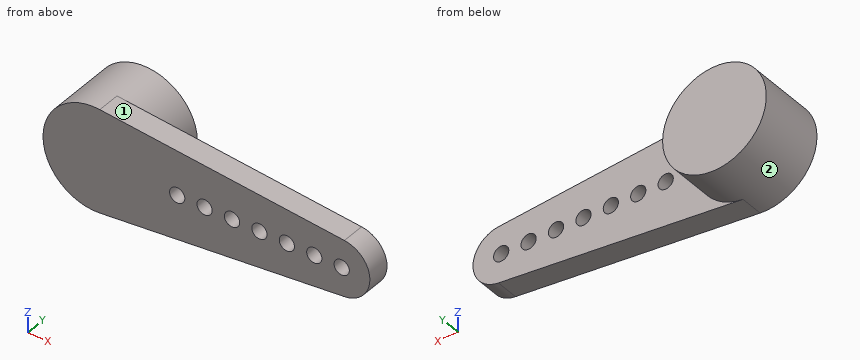
from build123d import *

# Parameters (mm, degrees)
SKETCH_1_R          = 3.405
EXTRUDE_1_DEPTH     = 4.5
EXTRUDE_2_DEPTH     = 1.52
SKETCH_3_R          = 0.5
CUT_EXTRUDE_1_DEPTH = 1.52


with BuildPart() as part:
    # 草图1 → 凸台-拉伸1 (new body)
    with BuildSketch(Plane(origin=(0, 0, 0), x_dir=(1, 0, 0), z_dir=(0, 1, 0))):
        Circle(SKETCH_1_R)
    extrude(amount=EXTRUDE_1_DEPTH)

    # 草图2 → 凸台-拉伸2 (add)
    with BuildSketch(Plane.XZ):
        with BuildLine():
            Line((0.326737118, 3.389287219), (16.38252237, 1.841462953))
            ThreePointArc((16.38252237, 1.841462953), (18.055, 0), (16.38252237, -1.841462953))
            Line((16.38252237, -1.841462953), (0.326737118, -3.389287219))
            ThreePointArc((0.326737118, -3.389287219), (-3.405, 0), (0.326737118, 3.389287219))
        make_face()
    extrude(amount=-EXTRUDE_2_DEPTH)

    # 草图3 → 切除-拉伸1 (cut)
    with BuildSketch(Plane.XZ):
        with Locations((16.205, 0)):
            Circle(SKETCH_3_R)
        with Locations((14.405, 0)):
            Circle(SKETCH_3_R)
        with Locations((12.605, 0)):
            Circle(SKETCH_3_R)
        with Locations((10.805, 0)):
            Circle(SKETCH_3_R)
        with Locations((9.005, 0)):
            Circle(SKETCH_3_R)
        with Locations((7.205, 0)):
            Circle(SKETCH_3_R)
        with Locations((5.405, 0)):
            Circle(SKETCH_3_R)
    extrude(amount=-CUT_EXTRUDE_1_DEPTH, mode=Mode.SUBTRACT)


solid = part.part
Read the model definition and answer for the solid it produces. Units are mm, in the model's axes. Face numbers are marked on the shaded views. A direction names the side the tool comes from. Coordinates: 2 decimals unless noted, no trailing zeros. Loops run counter-clockwise (first coordinate to the right, second up) from the corner with the lowest first, then second, coordinate; pieces in that order, holes last. Notation, with made-up numbers: (44.25, -5.5) -> (83.25, -5.5) arc R8 ccw to (83.25, 1.5) -> close; hole circle Ø8 at (80.25, 72.5). An arc over 180 degrees is marked (long way). Write item = value, one per line. Start each with the question number.
1) Find the intervals of material crossed by L1, parallel to Y at x = 4.25, z = -1.75; L2, parallel to Z at x = 16.25, y = 1.05; L3, parallel to Z at x = -0.5, y = 1.35, in increasing order. Write a range as from..to.
2) The part is cut by section A-A, the plane z = 0. State how many separate pieces and enclosed holes the cut face has, plus the area to 3 significant figures.
3) The part is cut by section C-C, the plane y = 3.25. Determine the outline of the cut face in (x, z) (3 decimals), plus the area to 3 significant figures.
4) The part is cut by section B-B, the plane y = 0.6. Determine the outline of the cut face in (x, z) (3 decimals).
5) For the marked faces 1 and 2, determine the directions among +Z, -Z, +X, -X, +Y, -Y from which every point of the face is accessible in a straight line to the end or side of a thin tool.
6) The part is cut by section D-D, the plane z = -1.5. Determine the outline of the cut face in (x, y), plus the area to 3 significant figures.
7) Given P1, Ø2, axis at x = 11, z = 0, coming from the +Y side; P2, Ø1.5, axis at x = 9, y = 1.5, coming from the -Z side, each flat-ended and moving along its own axis, determine where each tip first touches the part or whether it passes through.
Result:
q1.L1 = 0..1.52
q1.L2 = -1.85..-0.5, 0.5..1.85
q1.L3 = -3.37..3.37
q2.separate_pieces = 8
q2.enclosed_holes = 0
q2.area = 42.3 mm²
q3.outline = circle Ø6.81 at (0, 0)
q3.area = 36.4 mm²
q4.outline = (0.327, -3.389) -> (16.383, -1.841) arc R1.85 ccw to (16.383, 1.841) -> (0.327, 3.389) arc R3.405 ccw (long way) to start; hole circle Ø1 at (5.405, 0); hole circle Ø1 at (7.205, 0); hole circle Ø1 at (9.005, 0); hole circle Ø1 at (10.805, 0); hole circle Ø1 at (12.605, 0); hole circle Ø1 at (14.405, 0); hole circle Ø1 at (16.205, 0)
q5.face_1 = +Z, +X, +Y, -Y
q5.face_2 = +Y
q6.outline = (-3.06, 0) -> (17.29, 0) -> (17.29, 1.52) -> (3.06, 1.52) -> (3.06, 4.5) -> (-3.06, 4.5) -> close
q6.area = 49.1 mm²
q7.P1 = 1.52
q7.P2 = -2.63
